Job drawing, mm, ordinate dimensions from the low corner. One solid piece. A direction names the side the tool comes from. Round coordinates to 2 decimals unless told otherwise and drop trailing zeros. Loops run counter-clockwise (first coordinate to the right, second up) from the corner with the lowest first, then second, coordinate; pieces in that order, holes last.
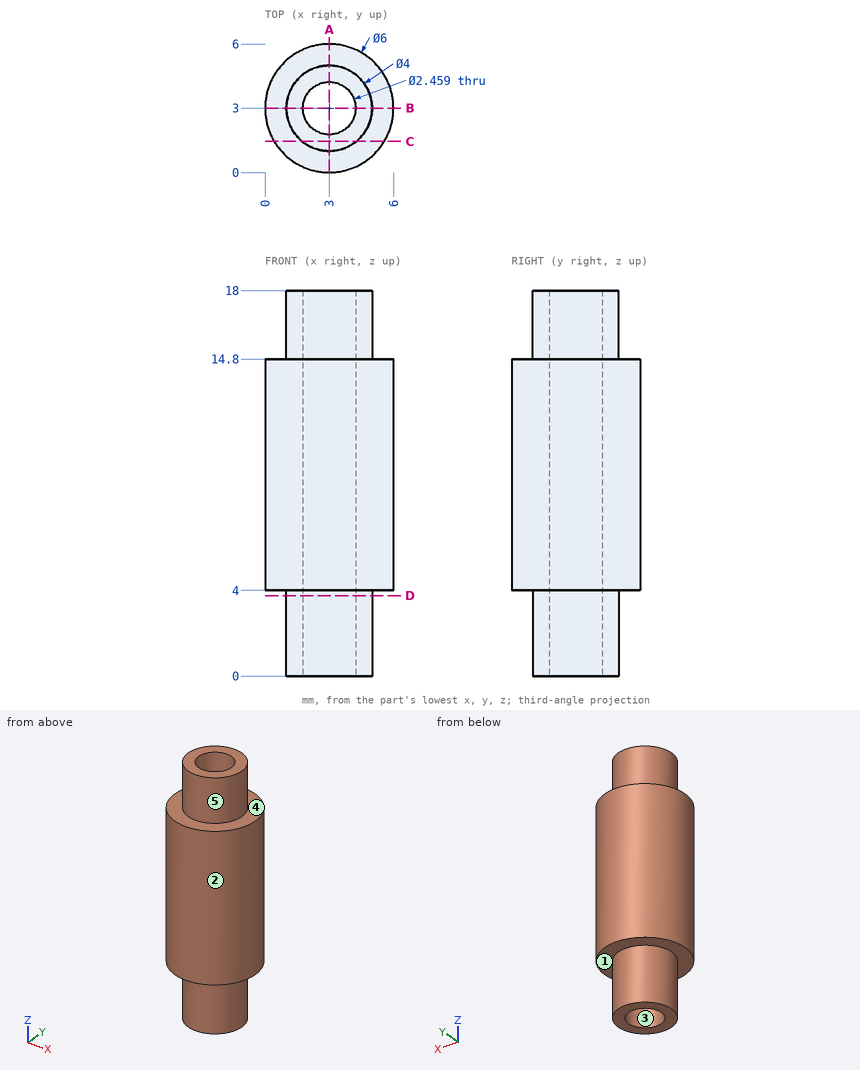
(1) Pull direction Y, two halves, no side cores. Call the marked faces 3, 4 and 5: +Y half, -Y half, draft (parallel to the pull), parting line (faces both ways), or undercut.
Responses:
face 3: undercut
face 4: draft
face 5: parting line
(2) Slice it at D-D on z = 3.75. List the corners of the cut face in (x, y).
Responses:
outline: circle Ø4 at (3, 3); hole circle Ø2.46 at (3, 3)
(3) Which spindle directions (+Z, -Z, +X, -X, +Y, -Y) get a long thin tool onto all of the face, cutting with end or side? Do the marked faces 1 and 2. Say none if no direction does.
Responses:
face 1: -Z
face 2: +Z, -Z
(4) Pin check, flat tips, straight feed: P1, Ø1.8, axis at x = 3, y = 2.5, coming from the +Z side; P2, Ø2, axis at x = 3, y = 3, coming from the -Z side (3 decimals). Stop position of each tip, or through.
Responses:
P1: stops at z = 18
P2: passes through
(5) Probe line 1 (Y direction, x = 3, z = 6.25); line 2 (Y direction, x = 2.95, z = 15.5); line 3 (X direction, y = 2.55, z = 7). List the from-to ranges inside material, lowest first.
Responses:
line 1: y = 0 to 1.77, 4.23 to 6
line 2: y = 1 to 1.77, 4.23 to 5
line 3: x = 0.03 to 1.86, 4.14 to 5.97
(6) Slice it at A-A on x = 3. List the corners of the cut face in (y, z), plus the area to 3 significant figures.
Responses:
outline: (0, 4) - (1, 4) - (1, 0) - (1.77, 0) - (1.77, 18) - (1, 18) - (1, 14.8) - (0, 14.8) - close; (4.23, 0) - (5, 0) - (5, 4) - (6, 4) - (6, 14.8) - (5, 14.8) - (5, 18) - (4.23, 18) - close
area: 49.3 mm2
(7) Slice it at C-C on y = 1.45. List the corners of the cut face in (x, z).
Responses:
outline: (0.43, 4) - (1.74, 4) - (1.74, 0) - (4.26, 0) - (4.26, 4) - (5.57, 4) - (5.57, 14.8) - (4.26, 14.8) - (4.26, 18) - (1.74, 18) - (1.74, 14.8) - (0.43, 14.8) - close
